Check sheet for the modelled part. Datum: model origin and axes. Units: mm. Face numbers are marked on the shaded views. A direction names the side the tool comes from. Give positions to 0.01 mm unless a question says otherwise; leave off trailing zeros. Order: outer loops, then holes, each group sorted by start corner. A loop starts at its lowest first (then second) coordinate and runs counter-clockwise, first axis right, second up.
Item 1: Sectioned sample at C-C on z = 60. Record the boundary of the cut face in (x, y).
Item 2: Material ranges on line 1 along Y through (x, z) = (-9.5, 24); line 2 along X through (y, z) = (19, 71); line 3 along Y through (x, z) = (10, 83), recorded low to high.
Item 3: Sectioned sample at A-A on x = -4. Record the boundary of the cut face in (y, z), and give its area (3 significant figures).
Item 4: Access from +Z, -Z, +X, -X, +Y, -Y to the whole of each face (thin tool, end or side, straight path). Record for the marked faces 4 and 5.
Item 5: Gauge pin test, flat end, axial feed: P1, Ø20, axis at x = -5.5, y = 13, coming from the -Z side. Record the tip position at first contact, or that the pin passes through.
Item 6: Sectioned sample at B-B on y = -6. Record the boundary of the cut face in (x, z).
Item 7: Release check for a two-part mould opening along X. For the marked faces 1, 2 and 3 record: released by +X, released by -X, zero draft, split by the parting line, or undercut.
Item 8: Sectioned sample at D-D on y = 11. Record the boundary of the cut face in (x, z), and give its area (3 significant figures).
from build123d import *

# Parameters (mm, degrees)
ESQUISSE1_W             = 61.5
ESQUISSE1_H             = 43.75
BOSS_EXTRU_1_DEPTH      = 88
ENL_V_MAT_EXTRU_4_REACH = 90
ESQUISSE3_W             = 53.5
ESQUISSE3_H             = 7.118224843
ESQUISSE6_W             = 57.502648101
ESQUISSE6_H             = 39.75
ENL_V_MAT_EXTRU_5_DEPTH = 82
CONG_4_R                = 2
ESQUISSE7_R             = 1.5
BOSS_EXTRU_2_DEPTH      = 5.2
ESQUISSE8_R             = 1.5
BOSS_EXTRU_3_DEPTH      = 5.2


with BuildPart() as part:
    # Esquisse1 → Boss.-Extru.1 (new body)
    with BuildSketch(Plane.XY):
        with Locations((-0.850502513, 12.751256281)):
            Rectangle(ESQUISSE1_W, ESQUISSE1_H)
    extrude(amount=BOSS_EXTRU_1_DEPTH)

    # Esquisse3 → Enlèv. mat.-Extru.4 (cut, up to next)
    with BuildSketch(Plane.XY.offset(88), mode=Mode.PRIVATE) as enl_v_mat_extru_4_sk1:
        with Locations((-0.850502513, -1.222513082)):
            Rectangle(ESQUISSE3_W, ESQUISSE3_H)
    enl_v_mat_extru_4_tool1 = extrude(enl_v_mat_extru_4_sk1.sketch, amount=-ENL_V_MAT_EXTRU_4_REACH, mode=Mode.PRIVATE) & part.part
    add(enl_v_mat_extru_4_tool1.solids().sort_by_distance((-0.850503, -1.222513, 88))[0], mode=Mode.SUBTRACT)

    # Esquisse6 → Enlèv. mat.-Extru.5 (cut)
    with BuildSketch(Plane(origin=(0, 0, 0), x_dir=(-1, 0, 0), z_dir=(0, 0, -1))):
        with Locations((0.849178462, 12.751256281)):
            Rectangle(ESQUISSE6_W, ESQUISSE6_H)
    extrude(amount=-ENL_V_MAT_EXTRU_5_DEPTH, mode=Mode.SUBTRACT)

    # Congé4
    cong_4_edges = [part.edges().sort_by_distance(p)[0] for p in [
        (29.899497487, 12.751256281, 88),
        (-0.850502513, 34.626256281, 88),
        (-31.600502513, 12.751256281, 88),
        (-31.600502513, 34.626256281, 44),
        (29.899497487, 34.626256281, 44),
        (29.899497487, -9.123743719, 44),
        (-31.600502513, -9.123743719, 44),
        (-0.850502513, -9.123743719, 88),
    ]]
    fillet(cong_4_edges, radius=CONG_4_R)

    # Esquisse7 → Boss.-Extru.2 (add)
    with BuildSketch(Plane(origin=(0, -7.123743719, 0), x_dir=(1, 0, 0), z_dir=(0, 1, 0))):
        with Locations((18.002145588, -9.4)):
            Circle(ESQUISSE7_R)
    extrude(amount=BOSS_EXTRU_2_DEPTH)

    # Esquisse8 → Boss.-Extru.3 (add)
    with BuildSketch(Plane(origin=(0, -7.123743719, 0), x_dir=(1, 0, 0), z_dir=(0, 1, 0))):
        with Locations((-9.850502513, -9.5)):
            Circle(ESQUISSE8_R)
    extrude(amount=BOSS_EXTRU_3_DEPTH)


solid = part.part
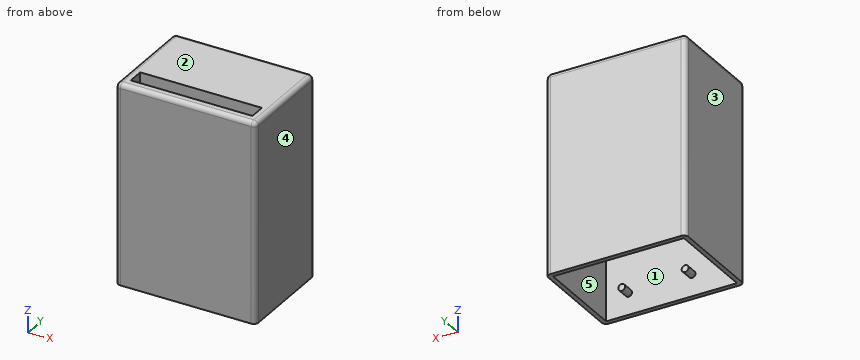
Report:
1. outline: (-31.6, -7.12) arc R2 ccw to (-29.6, -9.12) - (27.9, -9.12) arc R2 ccw to (29.9, -7.12) - (29.9, 32.63) arc R2 ccw to (27.9, 34.63) - (-29.6, 34.63) arc R2 ccw to (-31.6, 32.63) - close; hole (-29.6, -7.12) - (27.9, -7.12) - (27.9, 32.63) - (-29.6, 32.63) - close
2. line 1: y = -9.12 to -7.12, 32.63 to 34.63
2. line 2: x = -31.6 to -29.6, 27.9 to 29.9
2. line 3: y = -9.12 to -4.78, 2.34 to 34.63
3. outline: (-9.12, 0) - (-7.12, 0) - (-7.12, 82) - (-4.78, 82) - (-4.78, 88) - (-7.12, 88) arc R2 ccw to (-9.12, 86) - close; (2.34, 82) - (32.63, 82) - (32.63, 0) - (34.63, 0) - (34.63, 86) arc R2 ccw to (32.63, 88) - (2.34, 88) - close
3. area: 546 mm2
4. face 4: +Z, -Z, +X, +Y, -Y
4. face 5: -Z
5. P1: stops at z = 82
6. outline: (-31.6, 0) - (-29.6, 0) - (-29.6, 82) - (27.9, 82) - (27.9, 0) - (29.9, 0) - (29.9, 86) arc R2 ccw to (27.9, 88) - (-29.6, 88) arc R2 ccw to (-31.6, 86) - close; circle Ø3 at (-9.85, 9.5); circle Ø3 at (18, 9.4)
7. face 1: undercut
7. face 2: zero draft
7. face 3: released by -X
8. outline: (-31.6, 0) - (-29.6, 0) - (-29.6, 82) - (27.9, 82) - (27.9, 0) - (29.9, 0) - (29.9, 86) arc R2 ccw to (27.9, 88) - (-29.6, 88) arc R2 ccw to (-31.6, 86) - close
8. area: 695 mm2
